Could you check a few things on this model? Use its own coordinates, in mm. Round coordinates to 2 decimals unless told otherwise and drop trailing zeros. Loops run counter-clockwise (first coordinate to the right, second up) from the corner with the lowest first, then second, coordinate; pieces in that order, holes last.
from build123d import *

# Parameters (mm, degrees)
BOSS_EXTRUDE1_DEPTH = 4


with BuildPart() as part:
    # Sketch1 → Boss-Extrude1 (new body)
    with BuildSketch(Plane.XY):
        with BuildLine():
            Line((-96.35, 107.6), (-103.304951288, 107.6))
            ThreePointArc((-103.304951288, 107.6), (-104.01205807, 107.307106781), (-104.304951288, 106.6))
            Line((-104.304951288, 106.6), (-104.304951288, 101))
            ThreePointArc((-104.304951288, 101), (-104.01205807, 100.292893219), (-103.304951288, 100))
            Line((-103.304951288, 100), (-100, 100))
            Line((-100, 100), (-100, 95.9))
            Line((-100, 95.9), (-103.304951288, 95.9))
            ThreePointArc((-103.304951288, 95.9), (-104.01205807, 95.607106781), (-104.304951288, 94.9))
            Line((-104.304951288, 94.9), (-104.304951288, 88.809262274))
            ThreePointArc((-104.304951288, 88.809262274), (-104.228830821, 88.426578842), (-104.01205807, 88.102155493))
            Line((-104.01205807, 88.102155493), (-100, 84.090097423))
            Line((-100, 84.090097423), (84.090097423, -100))
            Line((84.090097423, -100), (88.102155493, -104.01205807))
            ThreePointArc((88.102155493, -104.01205807), (88.426578842, -104.228830821), (88.809262274, -104.304951288))
            Line((88.809262274, -104.304951288), (94.9, -104.304951288))
            ThreePointArc((94.9, -104.304951288), (95.607106781, -104.01205807), (95.9, -103.304951288))
            Line((95.9, -103.304951288), (95.9, -100))
            Line((95.9, -100), (100, -100))
            Line((100, -100), (100, -103.304951288))
            ThreePointArc((100, -103.304951288), (100.292893219, -104.01205807), (101, -104.304951288))
            Line((101, -104.304951288), (106.6, -104.304951288))
            ThreePointArc((106.6, -104.304951288), (107.307106781, -104.01205807), (107.6, -103.304951288))
            Line((107.6, -103.304951288), (107.6, -96.35))
            ThreePointArc((107.6, -96.35), (106.743644741, -92.044811386), (104.304951288, -88.395048712))
            Line((104.304951288, -88.395048712), (100, -84.090097423))
            Line((100, -84.090097423), (-84.090097423, 100))
            Line((-84.090097423, 100), (-88.395048712, 104.304951288))
            ThreePointArc((-88.395048712, 104.304951288), (-92.044811386, 106.743644741), (-96.35, 107.6))
        make_face()
    extrude(amount=BOSS_EXTRUDE1_DEPTH)


solid = part.part
Item 1: If we section it at A-A, the plane z = 2.65: Please give me the cut outline in (x, y).
Results list:
outline: (-104.3, 88.81) arc R1 ccw to (-104.01, 88.1) - (88.1, -104.01) arc R1 ccw to (88.81, -104.3) - (94.9, -104.3) arc R1 ccw to (95.9, -103.3) - (95.9, -100) - (100, -100) - (100, -103.3) arc R1 ccw to (101, -104.3) - (106.6, -104.3) arc R1 ccw to (107.6, -103.3) - (107.6, -96.35) arc R11.25 ccw to (104.3, -88.4) - (-88.4, 104.3) arc R11.25 ccw to (-96.35, 107.6) - (-103.3, 107.6) arc R1 ccw to (-104.3, 106.6) - (-104.3, 101) arc R1 ccw to (-103.3, 100) - (-100, 100) - (-100, 95.9) - (-103.3, 95.9) arc R1 ccw to (-104.3, 94.9) - close
Item 2: Will these pins go through, and if not, where does the flat tip stop? pin 1 (1 mm diameter, centred on y = -12.5, z = 3, fed in from -X); pin 2 (1 mm diameter, centred on y = -101, z = 1, fed in from -X); pin 3 (2 mm diameter, centred on y = -78.5, z = 1, fed in from -X).
Results list:
pin 1: stops at x = -3.91
pin 2: stops at x = 84.59
pin 3: stops at x = 61.59
Item 3: If we section it at C-C, the plane y = 9.5: Please give me the cut outline in (x, z).
Results list:
outline: (-25.41, 0) - (6.41, 0) - (6.41, 4) - (-25.41, 4) - close
Item 4: If I drill on line 1 along Y through (x, z) = (-82.5, 1.5); line 2 along X through (y, z) = (43.5, 2.4); line 3 along X through (y, z) = (24.5, 2.75), over which ranges is the centre line in solid material (lowest first)?
Results list:
line 1: y = 66.59 to 98.41
line 2: x = -59.41 to -27.59
line 3: x = -40.41 to -8.59
Item 5: If we section it at B-B, the plane x = 92: Please give me the cut outline in (y, z).
Results list:
outline: (-104.3, 0) - (-76.09, 0) - (-76.09, 4) - (-104.3, 4) - close
